Solid Edge part; units mm, degrees
sketch "Sketch1" plane through (0, 0, 0) normal (0, 0, 1) x (1, 0, 0)
  line L0 (3.5, 3.5) -> (-3.5, 3.5)
  line L1 (-3.5, 3.5) -> (-3.5, -3.5)
  line L2 (-3.5, -3.5) -> (3.5, -3.5)
  line L3 (3.5, -3.5) -> (3.5, 3.5)
  line L4 (5.6569, -2) -> (10, -2)
  line L5 (10, -2) -> (10, 2)
  line L6 (10, 2) -> (5.6569, 2)
  arc A0 (-5.6569, 2) -> (5.6569, 2) centre (0, 0) cw
  line L7 (-5.6569, 2) -> (-10, 2)
  line L8 (-10, 2) -> (-10, -2)
  line L9 (-10, -2) -> (-5.6569, -2)
  arc A1 (-5.6569, -2) -> (5.6569, -2) centre (0, 0) ccw
extrude "Protrusion1" add sketch "Sketch1" along normal blind 6
Can you work these out from the model? Positions are in its coordinate system, mm. A direction names the side the tool comes from. Round coordinates to 2 decimals unless told otherwise and drop trailing zeros. Loops run counter-clockwise (first coordinate to the right, second up) from the corner with the lowest first, then second, coordinate; pieces in that order, holes last. Notation, with made-up numbers: (62, -36) -> (104, -36) arc R19 ccw to (104, -18) -> close; hole circle Ø7 at (-5, -30.5). An arc over 180 degrees is marked (long way). Answer in a Markdown table with one row per item.
Item 1: We'd pull the mould along Y, two halves only. Please class faces 3 (the flat face through (-10, 0, 3)), 4 (the flat face through (3.5, 0, 3)), 5 (the cylindrical face through (0, -6, 3)), 6 (the cylindrical face through (0, 6, 3)): released by +Y, released by -Y, zero draft, split by the parting line, or undercut.
Answer block:
| item | result |
|---|---|
| face 3 | zero draft |
| face 4 | undercut |
| face 5 | released by -Y |
| face 6 | released by +Y |
Item 2: Suppose I cut it at C-C, the plane z = 2.5. List the corners of the cut face in (x, y) for me.
Answer block:
| item | result |
|---|---|
| outline | (-10, -2) -> (-5.66, -2) arc R6 ccw to (5.66, -2) -> (10, -2) -> (10, 2) -> (5.66, 2) arc R6 ccw to (-5.66, 2) -> (-10, 2) -> close; hole (-3.5, -3.5) -> (3.5, -3.5) -> (3.5, 3.5) -> (-3.5, 3.5) -> close |
Item 3: Suppose I cut it at B-B, the plane x = -2. List the corners of the cut face in (y, z) for me, plus the area to 3 significant figures.
Answer block:
| item | result |
|---|---|
| outline | (-5.66, 0) -> (-3.5, 0) -> (-3.5, 6) -> (-5.66, 6) -> close; (3.5, 0) -> (5.66, 0) -> (5.66, 6) -> (3.5, 6) -> close |
| area | 25.9 mm² |
Item 4: Suppose I cut it at D-D, the plane x = 7.5. List the corners of the cut face in (y, z) for me, plus the area to 3 significant figures.
Answer block:
| item | result |
|---|---|
| outline | (-2, 0) -> (2, 0) -> (2, 6) -> (-2, 6) -> close |
| area | 24.0 mm² |
Item 5: If I drill on probe 1 along Y at (x, z) = (2, 2.9); probe 2 along X at (y, z) = (0.5, 3.1); probe 3 along Y at (x, z) = (-8, 5.1), over which ranges is the centre line in solid material (lowest first)?
Answer block:
| item | result |
|---|---|
| probe 1 | -5.66 to -3.5, 3.5 to 5.66 |
| probe 2 | -10 to -3.5, 3.5 to 10 |
| probe 3 | -2 to 2 |
Item 6: Will these pins go through, and if not, where does the flat tip stop? P1, Ø1.3, axis at x = -8.5, z = 2.5, coming from the -Y side; P2, Ø3.5, axis at x = 7, z = 2, coming from the -Y side; P3, Ø2, axis at x = 7, z = 2, coming from the +Y side.
Answer block:
| item | result |
|---|---|
| P1 | y = -2 |
| P2 | y = -2.9 |
| P3 | y = 2 |
Item 7: On a 3-axis mill with a long thin cutter (end or side, diameter ignored), from which of +Z, -Z, +X, -X, +Y, -Y can I reach the whole of each face in a straight line? I mean faces 1 (the flat face through (0, -3.5, 3)), 2 (the flat face through (0, 4, 6)). Say none if no direction works.
Answer block:
| item | result |
|---|---|
| face 1 | +Z, -Z |
| face 2 | +Z, +X, -X, +Y, -Y |
Item 8: Suppose I cut it at A-A, the plane y = 0. List the corners of the cut face in (x, z) for me.
Answer block:
| item | result |
|---|---|
| outline | (-10, 0) -> (-3.5, 0) -> (-3.5, 6) -> (-10, 6) -> close; (3.5, 0) -> (10, 0) -> (10, 6) -> (3.5, 6) -> close |
